Build history of the part. All positions in model axes, mm. A direction names the side the tool comes from. Round coordinates to 2 decimals unless told otherwise and drop trailing zeros. Write each loop counter-clockwise with the first axis right and the second up, starting at its lowest first coordinate (ties: lowest second). Pieces come first, ordered by that corner, then holes.
from build123d import *

# Parameters (mm, degrees)
SKETCH1_W               = 40
SKETCH1_H               = 30
BOSS_EXTRUDE1_DEPTH     = 90
SHELL1_T                = -3
FILLET1_R               = 5
CUT_EXTRUDE1_DEPTH      = 94.407708461
CUT_EXTRUDE1_DEPTH_BACK = 94.407708461
CUT_EXTRUDE2_DEPTH      = 94.407708461
CUT_EXTRUDE2_DEPTH_BACK = 94.407708461
SKETCH3_W               = 17.5
SKETCH3_H               = 40
SKETCH5_W               = 2
SKETCH5_H               = 40
BOSS_EXTRUDE2_DEPTH     = 3
SKETCH6_W               = 2
SKETCH6_H               = 18
BOSS_EXTRUDE3_DEPTH     = 3
SKETCH8_W               = 50
SKETCH8_H               = 50
BOSS_EXTRUDE4_DEPTH     = 15
SKETCH10_W              = 45
SKETCH10_H              = 10
CUT_EXTRUDE4_DEPTH      = 37.5
BOSS_EXTRUDE5_REACH     = 103.861
SKETCH15_W              = 10
SKETCH15_H              = 10
CUT_EXTRUDE8_DEPTH      = 103.988587343
CUT_EXTRUDE8_DEPTH_BACK = 103.988587343
SKETCH20_R              = 2
SKETCH21_R              = 4
CUT_EXTRUDE9_DEPTH      = 5


with BuildPart() as part:
    # Sketch1 → Boss-Extrude1 (new body)
    with BuildSketch(Plane(origin=(0, 0, 0), x_dir=(1, 0, 0), z_dir=(0, 1, 0))):
        Rectangle(SKETCH1_W, SKETCH1_H)
    extrude(amount=BOSS_EXTRUDE1_DEPTH)

    # Shell1
    shell1_openings = [part.faces().sort_by_distance(p)[0] for p in [
        (0, 90, 0),
        (0, 0, 0),
    ]]
    offset(amount=SHELL1_T, openings=shell1_openings, kind=Kind.INTERSECTION)

    # Fillet1
    fillet1_edges = [part.edges().sort_by_distance(p)[0] for p in [
        (20, 45, 15),
        (-20, 45, 15),
        (-20, 45, -15),
        (20, 45, -15),
    ]]
    fillet(fillet1_edges, radius=FILLET1_R)

    # Sketch2 → Cut-Extrude1 (cut, two sides: drawn at the far end of the back side and taken through both)
    with BuildSketch(Plane.XY.offset(-CUT_EXTRUDE1_DEPTH_BACK)):
        Polygon((-5.5, 90), (-20, 66), (-20, 90), align=None)
    extrude(amount=CUT_EXTRUDE1_DEPTH + CUT_EXTRUDE1_DEPTH_BACK, mode=Mode.SUBTRACT)

    # Sketch3 → Cut-Extrude2 (cut, two sides: drawn at the far end of the back side and taken through both)
    with BuildSketch(Plane.XY.offset(-CUT_EXTRUDE2_DEPTH_BACK)):
        with Locations((11.25, 70)):
            Rectangle(SKETCH3_W, SKETCH3_H)
    extrude(amount=CUT_EXTRUDE2_DEPTH + CUT_EXTRUDE2_DEPTH_BACK, mode=Mode.SUBTRACT)

    # Sketch5 → Boss-Extrude2 (add)
    with BuildSketch(Plane(origin=(2.5, 0, 0), x_dir=(0, 0, -1), z_dir=(1, 0, 0))):
        with Locations((-13.5, 70)):
            Rectangle(SKETCH5_W, SKETCH5_H)
    boss_extrude2 = extrude(amount=BOSS_EXTRUDE2_DEPTH)

    # Mirror1: Boss-Extrude2 across plane
    add(boss_extrude2.mirror(Plane.XY))

    # Sketch6 → Boss-Extrude3 (add)
    with BuildSketch(Plane(origin=(-43.86391097, 26.501112878, 0), x_dir=(0, 0, 1), z_dir=(-0.8559155419457907, 0.5171156399255815, 0))):
        with Locations((-13.5, 65.188262756)):
            Rectangle(SKETCH6_W, SKETCH6_H)
    boss_extrude3 = extrude(amount=BOSS_EXTRUDE3_DEPTH)

    # Mirror2: Boss-Extrude3 across plane
    add(boss_extrude3.mirror(Plane.XY))

    # Sketch8 → Boss-Extrude4 (add)
    with BuildSketch(Plane(origin=(0, 0, 0), x_dir=(1, 0, 0), z_dir=(0, 1, 0))):
        Rectangle(SKETCH8_W, SKETCH8_H)
    extrude(amount=-BOSS_EXTRUDE4_DEPTH)

    # Sketch10 → Cut-Extrude4 (cut)
    with BuildSketch(Plane.ZY.offset(25)):
        with Locations((0, -7.5)):
            Rectangle(SKETCH10_W, SKETCH10_H)
    extrude(amount=-CUT_EXTRUDE4_DEPTH, mode=Mode.SUBTRACT)

    # Sketch15 → Boss-Extrude5 (add, up to next)
    with BuildSketch(Plane.XY.offset(-12), mode=Mode.PRIVATE) as boss_extrude5_sk1:
        with Locations((-12, 5)):
            Rectangle(SKETCH15_W, SKETCH15_H)
    boss_extrude5_tool1 = extrude(boss_extrude5_sk1.sketch, amount=BOSS_EXTRUDE5_REACH, mode=Mode.PRIVATE) - part.part
    add(boss_extrude5_tool1.solids().sort_by_distance((-12, 5, -12))[0])

    # Sketch20 → Cut-Extrude8 (cut, two sides: drawn at the far end of the back side and taken through both)
    with BuildSketch(Plane(origin=(0, 0, -15), x_dir=(-1, 0, 0), z_dir=(0, 0, -1)).offset(-CUT_EXTRUDE8_DEPTH_BACK)):
        with Locations((12, 5)):
            Circle(SKETCH20_R)
    extrude(amount=CUT_EXTRUDE8_DEPTH + CUT_EXTRUDE8_DEPTH_BACK, mode=Mode.SUBTRACT)

    # Sketch21 → Cut-Extrude9 (cut)
    with BuildSketch(Plane(origin=(0, 0, -15), x_dir=(-1, 0, 0), z_dir=(0, 0, -1))):
        with Locations((12, 5)):
            Circle(SKETCH21_R)
    cut_extrude9 = extrude(amount=-CUT_EXTRUDE9_DEPTH, mode=Mode.SUBTRACT)

    # Mirror3: Cut-Extrude9 across plane
    add(cut_extrude9.mirror(Plane.XY), mode=Mode.SUBTRACT)


solid = part.part
1) Pin check, flat tips, straight feed: pin 1 Ø9 at (x, z) = (13.5, 7) entering from +Y; pin 2 Ø12 at (y, z) = (34, -6) entering from -X; pin 3 Ø3 at (y, z) = (24.5, -10.5) entering from +X; pin 4 Ø3 at (x, y) = (-12, 5) entering from -Z. Stop position of each tip, or through.
Results:
pin 1: stops at y = 50
pin 2: stops at x = -20
pin 3: stops at x = 20
pin 4: passes through
2) Slice it at A-A (z = 3). Write the cut outline in (x, y).
Results:
outline: (-25, -15) - (25, -15) - (25, 0) - (20, 0) - (20, 50) - (17, 50) - (17, 0) - (-7, 0) - (-7, 10) - (-17, 10) - (-17, 70.97) - (-20, 66) - (-20, 0) - (-25, 0) - (-25, -2.5) - (12.5, -2.5) - (12.5, -12.5) - (-25, -12.5) - close; hole circle Ø4 at (-12, 5)
3) Slice it at D-D (y = 82). Write the cut outline in (x, z).
Results:
outline: (-13.84, -14.5) - (-10.33, -14.5) - (-10.33, -15) - (2.5, -15) - (2.5, -14.5) - (5.5, -14.5) - (5.5, -12.5) - (2.5, -12.5) - (2.5, -12) - (-10.33, -12) - (-10.33, -12.5) - (-13.84, -12.5) - close; (-13.84, 12.5) - (-10.33, 12.5) - (-10.33, 12) - (2.5, 12) - (2.5, 12.5) - (5.5, 12.5) - (5.5, 14.5) - (2.5, 14.5) - (2.5, 15) - (-10.33, 15) - (-10.33, 14.5) - (-13.84, 14.5) - close
4) Which spindle directions (+Z, -Z, +X, -X, +Y, -Y) get a long thin tool onto all of the face, cutting with end or side? Do faces 4 (the flat face through (0, 90, 13)), 5 (the flat face through (-12, 10, 0)), 6 (the flat face through (0, 34, -15)), 7 (the flat face through (-11, 83, 12.5)). Say none if no direction does.
Results:
face 4: +Z, -Z, +X, +Y
face 5: +Y
face 6: -Z, +X, -X, +Y
face 7: -X, +Y
5) Slice it at B-B (x = -22). Write the cut outline in (y, z).
Results:
outline: (-15, -25) - (0, -25) - (0, 25) - (-15, 25) - close; hole (-12.5, -22.5) - (-2.5, -22.5) - (-2.5, 22.5) - (-12.5, 22.5) - close
6) Mould opens along Y. For faces 1 (the flat face through (-6.766, 90.765, 13.514)), 2 (the flat face through (0, 34, -12)), 3 (the cylindrical face through (-8.8, 2.6, -12.5)) say: released by +Y, released by -Y, zero draft, split by the parting line, or undercut.
Results:
face 1: released by +Y
face 2: zero draft
face 3: undercut
7) Slice it at C-C (y = 5). Write the cut outline in (x, z).
Results:
outline: (-20, -10) arc R5 ccw to (-16, -14.9) - (-16, -10) - (-14, -10) - (-14, 10) - (-16, 10) - (-16, 14.9) arc R5 ccw to (-20, 10) - close; (-10, -10) - (-8, -10) - (-8, -15) - (15, -15) arc R5 ccw to (20, -10) - (20, 10) arc R5 ccw to (15, 15) - (-8, 15) - (-8, 10) - (-10, 10) - close; hole (-7, -12) - (17, -12) - (17, 12) - (-7, 12) - close
8) Wall check: L1, parallel to Y at x = -12, z = -5.5; L2, parallel to Y at x = -12, z = 11; L3, parallel to X at y = 5, z = 1.25. Give the ranges that are in metal, low to high.
Results:
L1: y = -15 to -12.5, -2.5 to 3, 7 to 10
L2: y = -15 to -12.5, -2.5 to 1, 9 to 10
L3: x = -20 to -14, -10 to -7, 17 to 20
